```python
from build123d import *

# Parameters (mm, degrees)
F1_DEPTH = 9.525
F2_R     = 2.5
F3_DEPTH = 1.901
F4_R     = 1.5
F5_DEPTH = 1.9
F6_R     = 7.5
F7_R     = 5


with BuildPart() as f1:
    # F0 (on Right) → F1 (new body, symmetric)
    with BuildSketch(Plane.YZ):
        with BuildLine():
            ThreePointArc((-3.1112698372, 7.5112698372), (-4.065069943, 2.7161928976), (0, 0))
            Line((0, 0), (50, 0))
            Line((50, 0), (50, 1.9))
            Line((50, 1.9), (0, 1.9))
            ThreePointArc((0, 1.9), (-2.3096988313, 3.4432914191), (-1.767766953, 6.167766953))
            Line((-1.767766953, 6.167766953), (15.9099025767, 23.8454364826))
            Line((15.9099025767, 23.8454364826), (14.5663996924, 25.1889393669))
            Line((14.5663996924, 25.1889393669), (-3.1112698372, 7.5112698372))
        make_face()
    extrude(amount=F1_DEPTH, both=True)

    # F2 (on face) → F3 (cut, through all)
    with BuildSketch(Plane.XY.offset(1.9)):
        with Locations((0, 18)):
            Circle(F2_R)
        with BuildLine():
            Line((2.5, 31.7094863951), (2.5, 41.7094863951))
            ThreePointArc((2.5, 41.7094863951), (0, 44.2094863951), (-2.5, 41.7094863951))
            Line((-2.5, 41.7094863951), (-2.5, 31.7094863951))
            ThreePointArc((-2.5, 31.7094863951), (0, 29.2094863951), (2.5, 31.7094863951))
        make_face()
    extrude(amount=-F3_DEPTH, mode=Mode.SUBTRACT)

    # F4 (on face) → F5 (cut)
    with BuildSketch(Plane(origin=(0, -5.3112698372, 5.3112698372), x_dir=(1, 0, 0), z_dir=(0, -0.7071067812, 0.7071067812))):
        with Locations((-5.025, 20.6112698372)):
            Circle(F4_R)
        with Locations((5.025, 20.6112698372)):
            Circle(F4_R)
    extrude(amount=-F5_DEPTH, mode=Mode.SUBTRACT)

    # F6
    f6_edges = [f1.edges().sort_by_distance(p)[0] for p in [
        (9.525, 15.238151, 24.517188),
        (-9.525, 15.238151, 24.517188),
    ]]
    fillet(f6_edges, radius=F6_R)

    # F7
    f7_edges = [f1.edges().sort_by_distance(p)[0] for p in [
        (-9.525, 50, 0.95),
        (9.525, 50, 0.95),
    ]]
    fillet(f7_edges, radius=F7_R)


solid = f1.part
```
Check sheet for the modelled part. Datum: model origin and axes. Units: mm. A direction names the side the tool comes from. Give positions to 0.01 mm unless a question says otherwise; leave off trailing zeros. Loops run counter-clockwise (first coordinate to the right, second up) from the corner with the lowest first, then second, coordinate; pieces in that order, holes last. Notation, with made-up numbers: M 0,82 L 44,82 A24 ccw 44,106 Z; hole C 51,38 d1. An arc over 180 degrees is marked long. Answer as CSV lines item,"result".
Item 1: Set-up check for faces 5 (the face through (-2.5, 37, 1)), 6 (the face through (0.133, 6.947, 14.883)), 7 (the face through (-0.33, 20.48, 0.96)), 8 (the face through (8.021, 48.574, 0.963)): record each of +Z, -Z, +X, -X, +Y, -Y from which the full face is reachable in a straight line by a thin tool's end or side.
Reply:
face 5,"+Z, -Z"
face 6,"+X, -X, +Y"
face 7,"-Z"
face 8,"+Z, -Z, +X, +Y"
Item 2: Draft check along Y on faces 1 (the face through (-5.35, 8.89, 18.19)), 2 (the face through (0.1, -4.1, 2.8)), 3 (the face through (-7.39, 13.63, 22.93)), 4 (the face through (-9.525, 15, 1)). Enter one of: pulls with the +Y half, pulls with the -Y half, needs draft (parallel to the pull), parting line crosses it, or undercut.
Reply:
face 1,"undercut"
face 2,"pulls with the -Y half"
face 3,"pulls with the +Y half"
face 4,"needs draft"
Item 3: Sectioned sample at B-B, the plane x = 0. Enter the section's corners in (y, z), then the cut area to 3 significant figures.
Reply:
outline,"M -3.11,7.51 A4.4 ccw 0,0 L 15.5,0 L 15.5,1.9 L 0,1.9 A2.5 cw -1.77,6.17 L 15.91,23.85 L 14.57,25.19 Z; M 20.5,0 L 29.21,0 L 29.21,1.9 L 20.5,1.9 Z; M 44.21,0 L 50,0 L 50,1.9 L 44.21,1.9 Z"
area,"120 mm^2"
Item 4: Sectioned sample at C-C, the plane x = 5.5. Enter the section's corners in (y, z), then the cut area to 3 significant figures.
Reply:
outline,"M -3.11,7.51 A4.4 ccw 0,0 L 49.9,0 L 49.9,1.9 L 0,1.9 A2.5 cw -1.77,6.17 L 9.6,17.54 L 8.26,18.88 Z; M 10.27,20.89 L 11.61,19.55 L 15.31,23.24 L 13.96,24.59 Z"
area,"151 mm^2"
Item 5: Sectioned sample at A-A, the plane y = 18. Enter the section's corners in (x, z) (3 decimals).
Reply:
outline,"M -9.525,0 L -2.5,0 L -2.5,1.9 L -9.525,1.9 Z; M 2.5,0 L 9.525,0 L 9.525,1.9 L 2.5,1.9 Z"
Item 6: Scan lines: L1, parallel to Y at x = 0, z = 1.35; L2, parallel to Y at x = 0, z = 1.05; L3, parallel to Z at x = 8, y = 29.5. Record each from-to range of solid material in increasing order.
Reply:
L1,"-3.17 to 15.5, 20.5 to 29.21, 44.21 to 50"
L2,"-2.85 to 15.5, 20.5 to 29.21, 44.21 to 50"
L3,"0 to 1.9"
Item 7: Depth check by flat-ended pin: pin 1 Ø1.5 at (y, z) = (27.5, 3.5) entering from +X; pin 2 Ø4.5 at (x, y) = (0, 18) entering from -Z; pin 3 Ø4 at (x, y) = (-7.5, 1.5) entering from -Z; pin 4 Ø10 at (x, z) = (-1.5, 10.5) entering from +Y. Enter the tip coordinate at first touch or a pass-through.
Reply:
pin 1,"through"
pin 2,"z = 23.69"
pin 3,"z = 0"
pin 4,"y = 7.56"
Item 8: Sectioned sample at D-D, the plane y = 2. Enter the section's corners in (x, z) (3 decimals), then the cut area to 3 significant figures.
Reply:
outline,"M -9.525,0 L 9.525,0 L 9.525,1.9 L -9.525,1.9 Z; M -9.525,9.936 L 9.525,9.936 L 9.525,12.623 L -9.525,12.623 Z"
area,"87.4 mm^2"
